CAD build for the part. Positions are in the model's coordinates, mm. A direction names the side the tool comes from. Round coordinates to 2 decimals unless told otherwise and drop trailing zeros. Write each loop counter-clockwise with the first axis right and the second up, starting at its lowest first coordinate (ties: lowest second). Pieces come first, ordered by that corner, then holes. Notation, with made-up numbers: (80.5, 36.25) - (84.5, 36.25) arc R27 ccw to (84.5, 57.25) - close; hole circle Ø10 at (88.5, 75). An arc over 180 degrees is marked (long way). Put each result on its own line as item: value. Start each with the question number.
Item 1: Cut at A-A (y = -160.5). Give the cut face in (x, z), and give its area (3 significant figures).
Item 2: Cut at C-C (x = -19). Give the cut face in (y, z).
Item 3: 3-axis set-ups, long thin cutter, end or side, ignore diameter. For faces 1 (the flat face through (-29, -175, -29.345)), 2 (the flat face through (-31, -175, -32.52)): which of +Z, -Z, +X, -X, +Y, -Y reach the whole face in a straight line?
Item 4: Cut at B-B (z = -26). Give the cut face in (x, y), and give its area (3 significant figures).
Item 5: Pin check, flat tips, straight feed: pin 1 Ø5 at (y, z) = (-208.5, 3) entering from +X; pin 2 Ø20.5 at (x, y) = (-29, -247) entering from +Z; pin 3 Ø1 at (x, z) = (-48, -23) entering from +Y. Stop position of each tip, or through.
Item 6: Drill centre lines: line 1 (X direction, y = -312, z = -24.5); line 2 (Z direction, x = -36.5, y = -291.5). Where is each one in solid material? Low to high. Write a range as from..to.
```python
from build123d import *

# Parameters (mm, degrees)
F1_DEPTH = 355.6
F3_DEPTH = 25.4
F5_DEPTH = 25.4


with BuildPart() as f1:
    # F0 (on Front) → F1 (new body)
    with BuildSketch(Plane.XZ):
        Polygon((-53.348197, 11.929806), (-53.348197, -32.520194), (-8.898197, -32.520194), (-8.898197, -29.345194), (-50.173197, -29.345194), (-50.173197, 11.929806), align=None)
    extrude(amount=F1_DEPTH)

    # F2 (on face) → F3 (cut)
    with BuildSketch(Plane.XY.offset(-29.345194)):
        Polygon((-50.173197, 0), (-8.898197, -41.275), (-8.898197, 0), align=None)
    extrude(amount=-F3_DEPTH, mode=Mode.SUBTRACT)

    # F4 (on face) → F5 (cut)
    with BuildSketch(Plane.XY.offset(-29.345194)):
        Polygon((-8.898197, -355.6), (-8.898197, -314.325), (-50.173197, -355.6), align=None)
    extrude(amount=-F5_DEPTH, mode=Mode.SUBTRACT)


solid = f1.part
```
Output values:
1. outline: (-53.35, -32.52) - (-8.9, -32.52) - (-8.9, -29.35) - (-50.17, -29.35) - (-50.17, 11.93) - (-53.35, 11.93) - close
1. area: 272 mm2
2. outline: (-324.43, -32.52) - (-31.17, -32.52) - (-31.17, -29.35) - (-324.43, -29.35) - close
3. face 1: +Z, +X, +Y, -Y
3. face 2: -Z, +X, -X, +Y, -Y
4. outline: (-53.35, -355.6) - (-50.17, -355.6) - (-50.17, 0) - (-53.35, 0) - close
4. area: 1,130 mm2
5. pin 1: x = -50.17
5. pin 2: z = -29.35
5. pin 3: through
6. line 1: -53.35..-50.17
6. line 2: -32.52..-29.35
